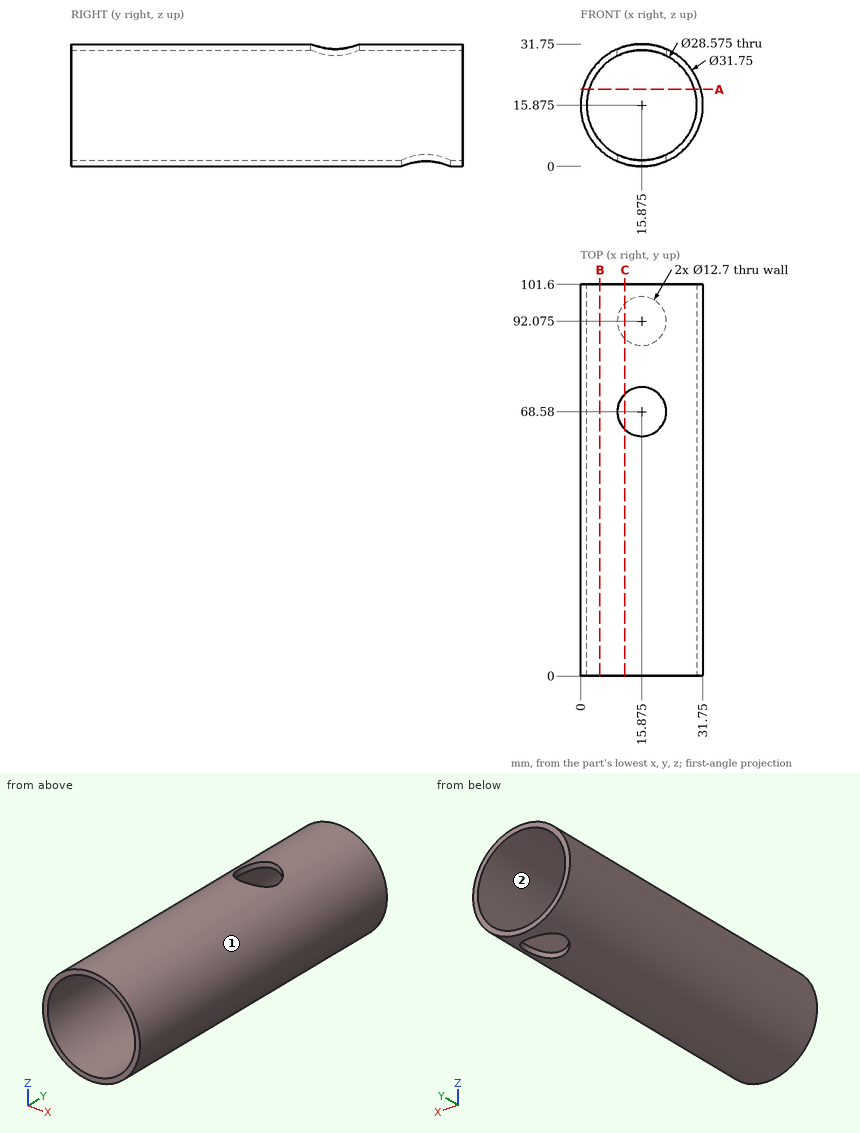
Design review of the part shown in the three views and the two pictorial views. Dimensions are in mm from the part's minimum x, y and z. Give positions to 0.01 mm unless a question says otherwise; leave off trailing zeros. Loops run counter-clockwise (first coordinate to the right, second up) from the corner with the lowest first, then second, coordinate; pieces in that order, holes last. Notation, with made-up numbers: (37.5, -4) - (60.5, -4) arc R19 ccw to (60.5, 15) - close; hole circle Ø1 at (56, 7.25). An arc over 180 degrees is marked (long way). Write item = value, one per line.
1) Take a section at A-A on z = 20. State the section outline as (x, y) points, and give its area (3 significant figures).
Result sheet:
outline = (0.55, 0) - (2.2, 0) - (2.2, 101.6) - (0.55, 101.6) - close; (29.55, 0) - (31.2, 0) - (31.2, 101.6) - (29.55, 101.6) - close
area = 335 mm2
2) Clearance check with flat-ended pins moving along their axes: pin 1 Ø10 at (x, y) = (21.5, 80) entering from -Z; pin 2 Ø3 at (x, y) = (10, 38.5) entering from +Z; pin 3 Ø6 at (y, z) = (24, 7.5) entering from -X. State where each tip first meets the part, or that it passes through.
Result sheet:
pin_1 = 0.01
pin_2 = 31.14
pin_3 = 0.94
3) Draft analysis for pull direction X (two halves, no side actions). For the marked faces 1 and 2, state which applies: +X half, -X half, draft (parallel to the pull), parting line (faces both ways), or undercut.
Result sheet:
face_1 = parting line
face_2 = undercut
4) To check wall thickness, follow line 1 (X direction, y = 83.5, z = 15.5); line 2 (X direction, y = 68, z = 30); line 3 (Z direction, x = 7, y = 31.5). State the ranges of each line that lie inside material, in increasing order.
Result sheet:
line_1 = 0 to 1.59, 30.16 to 31.75
line_2 = 8.63 to 9.55, 22.2 to 23.12
line_3 = 2.71 to 4.68, 27.07 to 29.04
5) Take a section at C-C on x = 11.5. State the section outline as (y, z) points.
Result sheet:
outline = (0, 0.61) - (87.47, 0.61) - (87.47, 2.27) - (0, 2.27) - close; (0, 29.48) - (63.98, 29.48) - (63.98, 31.14) - (0, 31.14) - close; (73.18, 29.48) - (101.6, 29.48) - (101.6, 31.14) - (73.18, 31.14) - close; (96.68, 0.61) - (101.6, 0.61) - (101.6, 2.27) - (96.68, 2.27) - close
6) Take a section at B-B on x = 5. State the section outline as (y, z) points, and give its area (3 significant figures).
Result sheet:
outline = (0, 4.31) - (101.6, 4.31) - (101.6, 6.61) - (0, 6.61) - close; (0, 25.14) - (101.6, 25.14) - (101.6, 27.44) - (0, 27.44) - close
area = 467 mm2
